```python
from build123d import *
from build123d.topology import SkipClean

# Parameters (mm, degrees)
SKETCH_1_W           = 65
SKETCH_1_H           = 65
EXTRUDE_1_DEPTH      = 17
CUT_EXTRUDE_1_DEPTH  = 59
CUT_EXTRUDE_2_DEPTH  = 79.260612028
EXTRUDE_2_DEPTH      = 10
SKETCH_12_W          = 35.24
SKETCH_12_H          = 8.5
CUT_EXTRUDE_5_DEPTH  = 79.260612028
SKETCH_17_R          = 2.25
CUT_EXTRUDE_8_DEPTH  = 58.965697588
EXTRUDE_START        = 10
SKETCH_18_W          = 65
SKETCH_18_H          = 65
SKETCH_18_R          = 2.25
EXTRUDE_3_DEPTH      = 10
CUT_EXTRUDE_START    = -10
SKETCH_9_R           = 11.25
SKETCH_9_R_2         = 10
CUT_EXTRUDE_3_DEPTH  = 5
CUT_EXTRUDE_START_2  = -20
SKETCH_10_R          = 11.25
SKETCH_10_R_2        = 10
CUT_EXTRUDE_4_DEPTH  = 5
SKETCH_19_W          = 65
SKETCH_19_H          = 6
CUT_EXTRUDE_9_DEPTH  = 17
SKETCH_20_W          = 65
SKETCH_20_H          = 6
CUT_EXTRUDE_10_DEPTH = 17
SKETCH_21_R          = 0.5
CUT_EXTRUDE_11_DEPTH = 69.629794564
CUT_EXTRUDE_12_DEPTH = 3.9
CUT_EXTRUDE_13_DEPTH = 60.168674963


with BuildPart() as part:
    # Эскиз1 → Бобышка-Вытянуть1 (new body)
    with BuildSketch(Plane(origin=(0, 0, 0), x_dir=(1, 0, 0), z_dir=(0, 1, 0))):
        with Locations((7.633818594, -8.451785088)):
            Rectangle(SKETCH_1_W, SKETCH_1_H)
    extrude(amount=EXTRUDE_1_DEPTH)

    # Эскиз3 → Вырез-Вытянуть1 (cut)
    with BuildSketch(Plane.XY.offset(37.951785088)):
        with BuildLine():
            Line((39.753818594, 8.5), (40.133818594, 8.5))
            Line((40.133818594, 8.5), (40.133818594, 0))
            Line((40.133818594, 0), (24.253818594, 0))
            Line((24.253818594, 0), (24.253818594, 8.5))
            ThreePointArc((24.253818594, 8.5), (32.003818594, 16.25), (39.753818594, 8.5))
        make_face()
        with BuildLine():
            Line((-24.486181406, 8.5), (-24.866181406, 8.5))
            Line((-24.866181406, 8.5), (-24.866181406, 0))
            Line((-24.866181406, 0), (-8.986181406, 0))
            Line((-8.986181406, 0), (-8.986181406, 8.5))
            ThreePointArc((-8.986181406, 8.5), (-16.736181406, 16.25), (-24.486181406, 8.5))
        make_face()
    extrude(amount=-CUT_EXTRUDE_1_DEPTH, mode=Mode.SUBTRACT)

    # Эскиз5 → Вырез-Вытянуть2 (cut, through all)
    with BuildSketch(Plane.XY.offset(40.951785088)):
        with BuildLine():
            Line((-23.486181406, 8.5), (-24.866181406, 8.5))
            Line((-24.866181406, 8.5), (-24.866181406, 0))
            Line((-24.866181406, 0), (-9.986181406, 0))
            Line((-9.986181406, 0), (-9.986181406, 8.5))
            ThreePointArc((-9.986181406, 8.5), (-16.736181406, 15.25), (-23.486181406, 8.5))
        make_face()
        with BuildLine():
            Line((38.753818594, 8.5), (40.133818594, 8.5))
            Line((40.133818594, 8.5), (40.133818594, 0))
            Line((40.133818594, 0), (25.253818594, 0))
            Line((25.253818594, 0), (25.253818594, 8.5))
            ThreePointArc((25.253818594, 8.5), (32.003818594, 15.25), (38.753818594, 8.5))
        make_face()
    extrude(amount=-CUT_EXTRUDE_2_DEPTH, mode=Mode.SUBTRACT)

    # Эскиз6 → Бобышка-Вытянуть2 (add)
    with BuildSketch(Plane.XY.offset(13.451785088)):
        with BuildLine():
            Line((-23.486181406, 8.5), (-24.866181406, 8.5))
            Line((-24.866181406, 8.5), (-24.866181406, 17))
            Line((-24.866181406, 17), (-9.986181406, 17))
            Line((-9.986181406, 17), (40.133818594, 17))
            Line((40.133818594, 17), (40.133818594, 8.5))
            Line((40.133818594, 8.5), (38.753818594, 8.5))
            ThreePointArc((38.753818594, 8.5), (32.003818594, 15.25), (25.253818594, 8.5))
            Line((25.253818594, 8.5), (25.253818594, 0))
            Line((25.253818594, 0), (-9.986181406, 0))
            Line((-9.986181406, 0), (-9.986181406, 8.5))
            ThreePointArc((-9.986181406, 8.5), (-16.736181406, 15.25), (-23.486181406, 8.5))
        make_face()
    extrude(amount=-EXTRUDE_2_DEPTH)

    # Эскиз12 → Вырез-Вытянуть5 (cut, through all)
    with BuildSketch(Plane.XY.offset(40.951785088)):
        with Locations((7.633818594, 4.25)):
            Rectangle(SKETCH_12_W, SKETCH_12_H)
    extrude(amount=-CUT_EXTRUDE_5_DEPTH, mode=Mode.SUBTRACT)

    # Эскиз17 → Вырез-Вытянуть8 (cut, through all)
    with BuildSketch(Plane(origin=(0, 17, 0), x_dir=(1, 0, 0), z_dir=(0, 1, 0))):
        with Locations(Location((7.633818594, 16.168732948, 0), (0, 0, 270))):
            Circle(SKETCH_17_R)
        with Locations(Location((7.676184998, -32.831267052, 0), (0, 0, 270))):
            Circle(SKETCH_17_R)
    extrude(amount=-CUT_EXTRUDE_8_DEPTH, mode=Mode.SUBTRACT)

    # Эскиз18 → Бобышка-Вытянуть3 (add)
    with BuildSketch(Plane(origin=(0, 17, 0), x_dir=(1, 0, 0), z_dir=(0, 1, 0)).offset(EXTRUDE_START)):
        with Locations((7.633818594, -8.451785088)):
            Rectangle(SKETCH_18_W, SKETCH_18_H)
        with Locations(Location((7.633818594, 16.168732948, 0), (0, 0, 270))):
            Circle(SKETCH_18_R, mode=Mode.SUBTRACT)
        with Locations(Location((7.676184998, -32.831267052, 0), (0, 0, 270))):
            Circle(SKETCH_18_R, mode=Mode.SUBTRACT)
    extrude(amount=-EXTRUDE_3_DEPTH)

    # Эскиз9 → Вырез-Вытянуть3 (cut)
    # profile 1 of 2: a face of its own
    with BuildSketch(Plane.XY.offset(37.951785088).offset(CUT_EXTRUDE_START)):
        with Locations((-16.736181406, 8.5)):
            Circle(SKETCH_9_R)
        with Locations((-16.736181406, 8.5)):
            Circle(SKETCH_9_R_2, mode=Mode.SUBTRACT)
    # profile 2 of 2: a face of its own
    with BuildSketch(Plane.XY.offset(37.951785088).offset(CUT_EXTRUDE_START)):
        with Locations((32.003818594, 8.5)):
            Circle(SKETCH_9_R)
        with Locations((32.003818594, 8.5)):
            Circle(SKETCH_9_R_2, mode=Mode.SUBTRACT)
    extrude(amount=-CUT_EXTRUDE_3_DEPTH, mode=Mode.SUBTRACT)

    # Эскиз10 → Вырез-Вытянуть4 (cut)
    # profile 1 of 2: a face of its own
    with BuildSketch(Plane.XY.offset(13.451785088).offset(CUT_EXTRUDE_START_2)):
        with Locations((-16.736181406, 8.5)):
            Circle(SKETCH_10_R)
        with Locations((-16.736181406, 8.5)):
            Circle(SKETCH_10_R_2, mode=Mode.SUBTRACT)
    # profile 2 of 2: a face of its own
    with BuildSketch(Plane.XY.offset(13.451785088).offset(CUT_EXTRUDE_START_2)):
        with Locations((32.003818594, 8.5)):
            Circle(SKETCH_10_R)
        with Locations((32.003818594, 8.5)):
            Circle(SKETCH_10_R_2, mode=Mode.SUBTRACT)
    extrude(amount=-CUT_EXTRUDE_4_DEPTH, mode=Mode.SUBTRACT)

    # Эскиз19 → Вырез-Вытянуть9 (cut)
    with BuildSketch(Plane(origin=(40.133818594, 0, 0), x_dir=(0, 0, -1), z_dir=(1, 0, 0))):
        with Locations((-8.451785088, 24)):
            Rectangle(SKETCH_19_W, SKETCH_19_H)
    extrude(amount=-CUT_EXTRUDE_9_DEPTH, mode=Mode.SUBTRACT)

    # Эскиз20 → Вырез-Вытянуть10 (cut)
    with BuildSketch(Plane.ZY.offset(24.866181406)):
        with Locations((8.451785088, 24)):
            Rectangle(SKETCH_20_W, SKETCH_20_H)
    extrude(amount=-CUT_EXTRUDE_10_DEPTH, mode=Mode.SUBTRACT)

    # Эскиз21 → Вырез-Вытянуть11 (cut, through all)
    with BuildSketch(Plane(origin=(23.133818594, 0, 0), x_dir=(0, 0, -1), z_dir=(1, 0, 0))):
        with Locations((-18.451785088, 24)):
            Circle(SKETCH_21_R)
        with Locations((1.548214912, 24)):
            Circle(SKETCH_21_R)
    extrude(amount=-CUT_EXTRUDE_11_DEPTH, mode=Mode.SUBTRACT)

    # Эскиз13 → Вырез-Вытянуть12 (cut)
    with BuildSketch(Plane.XZ.offset(-27)):
        with BuildLine():
            ThreePointArc((2.962122683, 12.40744876), (7.675512515, 2.131407246), (12.250269981, 12.469911346))
            ThreePointArc((12.250269981, 12.469911346), (7.501160594, 28.057428262), (2.962122683, 12.40744876))
        make_face()
    extrude(amount=CUT_EXTRUDE_12_DEPTH, mode=Mode.SUBTRACT)

    # Эскиз24 → Вырез-Вытянуть13 (cut, through all)
    with SkipClean():  # the faces are left unmerged after this step: merging them gives an invalid solid
        with BuildSketch(Plane(origin=(0, 23.1, 0), x_dir=(1, 0, 0), z_dir=(0, 1, 0))):
            with BuildLine():
                ThreePointArc((-0.190214084, -16.063311585), (7.501160594, -28.057428262), (15.353152659, -16.167840384))
                ThreePointArc((15.353152659, -16.167840384), (7.707791679, 2.668484217), (-0.190214084, -16.063311585))
            make_face()
        extrude(amount=-CUT_EXTRUDE_13_DEPTH, mode=Mode.SUBTRACT)


solid = part.part
```
The listing builds one solid part. Answer for the finished solid, in the listing's coordinates (mm). A direction names the side the tool comes from. Give positions to 0.01 mm unless a question says otherwise; leave off trailing zeros. Order: outer loops, then holes, each group sorted by start corner. A loop starts at its lowest first (then second) coordinate and runs counter-clockwise, first axis right, second up. Notation, with made-up numbers: (80, 87.5) -> (85, 87.5) arc R10 ccw to (85, 101.5) -> close; hole circle Ø5 at (-15.75, -3.5). An arc over 180 degrees is marked (long way). Answer as CSV lines item,"result". Start each with the question number.
Q1. Determine the mould class of faces 1 (the flat face through (28, 18, -6.548)), 2 (the cylindrical face through (27.99, 19.01, 25.49)), 3 (the cylindrical face through (31.83, 16.25, 25.87)), 4 (the flat face through (32, 16, 3.452)) for opening direction Y: pulls with the +Y half, pulls with the -Y half, needs draft (parallel to the pull), parting line crosses it, or undercut.
Q2. A cutting plane is placed at C-C (x = 35). Determine the outline of the cut face in (y, z).
Q3. Given pin 1 (13.5 mm diameter, centred on x = 34.5, z = 11, fed in from +Y); pin 2 (1.8 mm diameter, centred on y = 23.5, z = 3, fed in from +X), each flat-ended and moving along its own axis, determine where each tip first touches the part or whether it passes through.
Q4. A cutting plane is placed at B-B (y = 10.25). Count the separate pieces of the cut face and the enclosed holes in it, then the cut area to 3 significant figures.
Q5. Find the intervals of material crossed by L1, parallel to Z at x = -7, y = 12.25; L2, parallel to X at y = 12, z = -3; L3, parallel to X at y = 15.25, z = 34.5, in increasing order.
Q6. A cutting plane is placed at D-D (z = -9). Determine the outline of the cut face in (x, y), then the cut area to 3 significant figures.
Q7. Which of the six approach directions +Z, -Z, +X, -X, +Y, -Y give full straight-line access (tool end or side, diameter ignored) to faces 5 (the flat face through (32, 21, 9)), 6 (the cylindrical face through (-13.511, 17.966, 25.487)), 7 (the flat face through (32, 16, -21.048))?
Q8. A cutting plane is placed at A-A (z = 24.5). Determine the outline of the cut face in (x, y), then the cut area to 3 significant figures.
Results found:
1,face 1,"undercut"
1,face 2,"undercut"
1,face 3,"pulls with the -Y half"
1,face 4,"needs draft"
2,outline,"(14.55, -24.05) -> (21, -24.05) -> (21, 40.95) -> (14.55, 40.95) -> (14.55, 37.95) -> (15.65, 37.95) -> (15.65, 13.45) -> (14.55, 13.45) -> (14.55, 3.45) -> (15.65, 3.45) -> (15.65, -21.05) -> (14.55, -21.05) -> close; hole (18.04, -11.55) -> (19.34, -11.55) -> (19.34, -6.55) -> (18.04, -6.55) -> close; hole (18.04, 22.95) -> (19.34, 22.95) -> (19.34, 27.95) -> (18.04, 27.95) -> close"
3,pin 1,"y = 21"
3,pin 2,"x = 23.13"
4,separate pieces,"3"
4,enclosed holes,"7"
4,area,"1,750 mm2"
5,L1,"-24.05 to -11.55, -6.55 to 22.95, 27.95 to 40.95"
5,L2,"-24.87 to -23.65, -9.82 to 25.09, 38.92 to 40.13"
5,L3,"-24.87 to -20.54, -12.93 to 6.17, 9.19 to 28.2, 35.81 to 40.13"
6,outline,"(-24.87, 8.5) -> (-24.49, 8.5) arc R7.75 cw to (-8.99, 8.5) -> (-6.74, 8.5) arc R10 ccw to (-24.87, 14.32) -> close; (-24.87, 16.28) arc R11.25 cw to (-5.49, 8.5) -> (20.75, 8.5) arc R11.25 cw to (40.13, 16.28) -> (40.13, 21) -> (23.13, 21) -> (23.13, 27) -> (-7.87, 27) -> (-7.87, 21) -> (-24.87, 21) -> close; (22, 8.5) -> (24.25, 8.5) arc R7.75 cw to (39.75, 8.5) -> (40.13, 8.5) -> (40.13, 14.32) arc R10 ccw to start"
6,area,"745 mm2"
7,face 5,"+Z, -Z, +X, +Y"
7,face 6,"none"
7,face 7,"-Y"
8,outline,"(-24.87, 8.5) -> (-24.49, 8.5) arc R7.75 cw to (-8.99, 8.5) -> (-6.74, 8.5) arc R10 ccw to (-24.87, 14.32) -> close; (-24.87, 16.28) arc R11.25 cw to (-5.49, 8.5) -> (0.64, 8.5) -> (0.64, 27) -> (-7.87, 27) -> (-7.87, 21) -> (-24.87, 21) -> close; (14.47, 8.5) -> (20.75, 8.5) arc R11.25 cw to (40.13, 16.28) -> (40.13, 21) -> (23.13, 21) -> (23.13, 27) -> (14.47, 27) -> close; (22, 8.5) -> (24.25, 8.5) arc R7.75 cw to (39.75, 8.5) -> (40.13, 8.5) -> (40.13, 14.32) arc R10 ccw to start"
8,area,"489 mm2"
